from build123d import *

# Parameters (mm, degrees)
SKETCH1_R           = 2.55
BOSS_EXTRUDE1_DEPTH = 2.25


with BuildPart() as part:
    # Sketch1 → Boss-Extrude1 (new body)
    with BuildSketch(Plane(origin=(0, 0, 0), x_dir=(1, 0, 0), z_dir=(0, 1, 0))):
        with BuildLine():
            Line((-61, 9), (61, 9))
            ThreePointArc((61, 9), (70, 0), (61, -9))
            Line((61, -9), (-61, -9))
            ThreePointArc((-61, -9), (-70, 0), (-61, 9))
        make_face()
        with Locations(Location((-10, 0, 0), (0, 0, 270))):
            Circle(SKETCH1_R, mode=Mode.SUBTRACT)
        with BuildLine():
            Line((-61, 2.6), (-30.85, 2.6))
            ThreePointArc((-30.85, 2.6), (-28.25, 0), (-30.85, -2.6))
            Line((-30.85, -2.6), (-61, -2.6))
            ThreePointArc((-61, -2.6), (-63.6, 0), (-61, 2.6))
        make_face(mode=Mode.SUBTRACT)
        with BuildLine():
            Line((61, -2.6), (30.85, -2.6))
            ThreePointArc((30.85, -2.6), (28.25, 0), (30.85, 2.6))
            Line((30.85, 2.6), (61, 2.6))
            ThreePointArc((61, 2.6), (63.6, 0), (61, -2.6))
        make_face(mode=Mode.SUBTRACT)
    extrude(amount=BOSS_EXTRUDE1_DEPTH)


solid = part.part
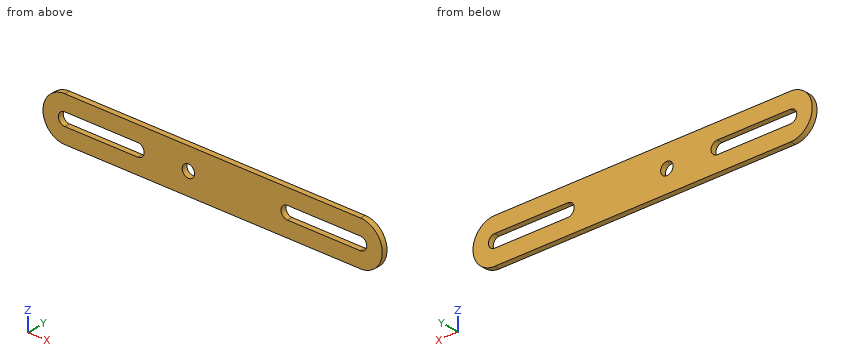
Could you check a few things on this model? Use its own coordinates, in mm. Give positions to 0.01 mm unless a question says otherwise; leave off trailing zeros. Order: outer loops, then holes, each group sorted by start corner. A loop starts at its lowest first (then second) coordinate and runs counter-clockwise, first axis right, second up. Notation, with made-up numbers: M 1.5,-0.5 L 15.5,-0.5 A31 ccw 15.5,23.5 Z; hole C -11.5,48 d9. An arc over 180 degrees is marked long. One line per question, with ' | ' between items.
1. If I drill on line 1 (X direction, y = 1.1, z = 0); line 2 (Z direction, x = -37, y = 0.15); line 3 (X direction, y = 0.75, z = 1), over which ranges is the centre line in solid material (lowest first)?
Results:
line 1: -70 to -63.6, -28.25 to -12.55, -7.45 to 28.25, 63.6 to 70 | line 2: -9 to -2.6, 2.6 to 9 | line 3: -69.94 to -63.4, -28.45 to -12.35, -7.65 to 28.45, 63.4 to 69.94
2. I want a section at B-B (z = 0). List the corners of the cut face in (x, y) for me, and give its area (3 significant figures).
Results:
outline: M -70,0 L -63.6,0 L -63.6,2.25 L -70,2.25 Z; M -28.25,0 L -12.55,0 L -12.55,2.25 L -28.25,2.25 Z; M -7.45,0 L 28.25,0 L 28.25,2.25 L -7.45,2.25 Z; M 63.6,0 L 70,0 L 70,2.25 L 63.6,2.25 Z | area: 144 mm²
3. I want a section at C-C (y = 0.85). List the corners of the cut face in (x, z) for me, and give its area (3 significant figures).
Results:
outline: M -61,-9 L 61,-9 A9 ccw 61,9 L -61,9 A9 ccw Z; hole M -61,-2.6 L -30.85,-2.6 A2.6 ccw -30.85,2.6 L -61,2.6 A2.6 ccw Z; hole C -10,0 d5.1; hole M 30.85,-2.6 L 61,-2.6 A2.6 ccw 61,2.6 L 30.85,2.6 A2.6 ccw Z | area: 2,070 mm²
4. I want a section at A-A (x = 46). List the corners of the cut face in (y, z) for me.
Results:
outline: M 0,-9 L 2.25,-9 L 2.25,-2.6 L 0,-2.6 Z; M 0,2.6 L 2.25,2.6 L 2.25,9 L 0,9 Z
